```python
from build123d import *

# Parameters (mm, degrees)
SKETCH1_R                                       = 84.5
SKETCH1_R_2                                     = 4.5
BOSS_EXTRUDE1_DEPTH                             = 10
SKETCH2_R                                       = 13
CUT_EXTRUDE1_DEPTH                              = 8
SKETCH3_R                                       = 12
BOSS_EXTRUDE2_DEPTH                             = 3
CIRPATTERN1_COUNT                               = 6
CSK_FOR_M2_FLAT_HEAD_MACHINE_SCREW1_D           = 2
CSK_FOR_M2_FLAT_HEAD_MACHINE_SCREW1_CSINK_D     = 4
CSK_FOR_M2_FLAT_HEAD_MACHINE_SCREW1_CSINK_ANGLE = 90
CIRPATTERN2_COUNT                               = 6


with BuildPart() as part:
    # Sketch1 → Boss-Extrude1 (new body)
    with BuildSketch(Plane.XY):
        Circle(SKETCH1_R)
        Circle(SKETCH1_R_2, mode=Mode.SUBTRACT)
    extrude(amount=BOSS_EXTRUDE1_DEPTH)

    # Sketch2 → Cut-Extrude1 (cut)
    with BuildSketch(Plane.XY):
        Circle(SKETCH2_R)
    extrude(amount=CUT_EXTRUDE1_DEPTH, mode=Mode.SUBTRACT)

    # Sketch3 → Boss-Extrude2 (add)
    with BuildSketch(Plane.XY.offset(10)):
        with Locations((84.204250337, 7.063584439)):
            Circle(SKETCH3_R)
    boss_extrude2 = extrude(amount=-BOSS_EXTRUDE2_DEPTH)

    # CirPattern1: Boss-Extrude2 ×6 about axis
    cirpattern1_axis = Axis((0, 0, 0), (0, 0, 1))
    for i in range(1, CIRPATTERN1_COUNT):
        add(boss_extrude2.rotate(cirpattern1_axis, i * 360 / CIRPATTERN1_COUNT))

    # CSK for M2 Flat Head Machine Screw1 (through all)
    with Locations(Plane(origin=(89.758705981, 7.529527266, 10), x_dir=(1, 0, 0), z_dir=(0, 0, 1))):
        with Locations((0, 0)):
            csk_for_m2_flat_head_machine_screw1 = CounterSinkHole(CSK_FOR_M2_FLAT_HEAD_MACHINE_SCREW1_D / 2, CSK_FOR_M2_FLAT_HEAD_MACHINE_SCREW1_CSINK_D / 2, counter_sink_angle=CSK_FOR_M2_FLAT_HEAD_MACHINE_SCREW1_CSINK_ANGLE)

    # CirPattern2: CSK for M2 Flat Head Machine Screw1 ×6 about axis
    cirpattern2_axis = Axis((0, 0, 0), (0, 0, 1))
    for i in range(1, CIRPATTERN2_COUNT):
        add(csk_for_m2_flat_head_machine_screw1.rotate(cirpattern2_axis, i * 360 / CIRPATTERN2_COUNT), mode=Mode.SUBTRACT)


solid = part.part
```
The listing builds one solid part. Answer for the finished solid, in the listing's coordinates (mm). A direction names the side the tool comes from. Round coordinates to 2 decimals unless told otherwise and drop trailing zeros. Loops run counter-clockwise (first coordinate to the right, second up) from the corner with the lowest first, then second, coordinate; pieces in that order, holes last. Notation, with made-up numbers: (23.25, 69.5) - (33.25, 69.5) arc R26 cw to (33.25, 101.5) - close; hole circle Ø7 at (14, 48). An arc over 180 degrees is marked (long way). Return JSON: item names as keys, results as strings. Group by question number.
1. Which of the six approach directions +Z, -Z, +X, -X, +Y, -Y give full straight-line access (tool end or side, diameter ignored) to faces 3 (the cylindrical face through (-54.84, 79.4, 8.52)), 4 (the flat face through (50, -72, 7)), 5 (the flat face through (-50, 72, 7)), 6 (the flat face through (38, 80, 7)), 7 (the flat face through (-38, -80, 7))?
2. The part is cut by section A-A on x = 0. Determine the outline of the cut face in (y, z), then the cut area to 3 significant figures.
3. Each of these flat-tipped pins is pushed along its axis until it touches: P1, Ø6, axis at y = 10, z = 7, coming from the -X side; P2, Ø4, axis at x = 87.5, y = 11.5, coming from the -Z side; P3, Ø10.5, axis at x = 0, y = 0, coming from the -Z side; P4, Ø1.8, axis at x = 51.4, y = -73.97, coming from the -Z side. Where does it stop, or does it pass through?
4. Consider probe 1 along Y at (x, z) = (0, 1.25); probe 2 along Y at (x, z) = (37, 1.25); probe 3 along X at (y, z) = (28.5, 6). Determine where each line is inside the solid, lowest interval first.
5. The mould has two halves that part along X. Classify faces 1 (the flat face through (-1, -18, 0)), 2 (the flat face through (6, 0, 8)): pulls with the +X half, pulls with the -X half, needs draft (parallel to the pull), parting line crosses it, or undercut.
6. The part is cut by section D-D on x = 34. Determine the outline of the cut face in (y, z), then the cut area to 3 significant figures.
7. The part is cut by section C-C on z = 2.75. Determine the outline of the cut face in (x, y).
8. The part is cut by section B-B on y = 0. Determine the outline of the cut face in (x, z), then the cut area to 3 significant figures.
Resolved:
{
 "1": {"face 3": "+Z, -Z", "face 4": "-Z, +X, -Y", "face 5": "-Z, -X, +Y", "face 6": "-Z, +X, +Y", "face 7": "-Z, -X, -Y"},
 "2": {"outline": "(-84.5, 0) - (-13, 0) - (-13, 8) - (-4.5, 8) - (-4.5, 10) - (-84.5, 10) - close; (4.5, 8) - (13, 8) - (13, 0) - (84.5, 0) - (84.5, 10) - (4.5, 10) - close", "area": "1,460 mm²"},
 "3": {"P1": "stops at x = -84.21", "P2": "stops at z = 7", "P3": "stops at z = 8", "P4": "passes through"},
 "4": {"probe 1": "y = -84.5 to -13, 13 to 84.5", "probe 2": "y = -75.97 to 75.97", "probe 3": "x = -79.55 to 79.55"},
 "5": {"face 1": "needs draft", "face 2": "undercut"},
 "6": {"outline": "(-77.36, 0) - (77.36, 0) - (77.36, 7) - (88.29, 7) - (88.29, 10) - (-77.36, 10) - close", "area": "1,580 mm²"},
 "7": {"outline": "circle Ø169 at (0, 0); hole circle Ø26 at (0, 0)"},
 "8": {"outline": "(-93.91, 7) - (-84.5, 7) - (-84.5, 0) - (-13, 0) - (-13, 8) - (-4.5, 8) - (-4.5, 10) - (-93.91, 10) - close; (4.5, 8) - (13, 8) - (13, 0) - (84.5, 0) - (84.5, 7) - (93.91, 7) - (93.91, 10) - (4.5, 10) - close", "area": "1,520 mm²"}
}
